Source: CAD feature listing. Evaluate the final solid. Frame: model axes, mm. Give positions to 0.01 mm unless a question says otherwise; leave off trailing zeros. Order: outer loops, then holes, each group sorted by start corner. A loop starts at its lowest first (then second) coordinate and runs counter-clockwise, first axis right, second up. Notation, with made-up numbers: M 69.5,62.25 L 126.5,62.25 A12 ccw 126.5,72.25 Z; hole C -26,52.5 d2. An arc over 180 degrees is marked long. Return JSON: item names as keys, results as strings.
from build123d import *

# Parameters (mm, degrees)
F0_W     = 266.7
F0_H     = 330.2
F1_DEPTH = 5.842
F2_W     = 266.7
F2_H     = 330.2
F2_W_2   = 215.9
F2_H_2   = 279.4
F3_DEPTH = 5.842
F6_R     = 9.525
F7_DEPTH = 11.685


with BuildPart() as f1:
    # F0 (on Front) → F1 (new body)
    with BuildSketch(Plane.XZ):
        with Locations((133.35, 165.1)):
            Rectangle(F0_W, F0_H)
    extrude(amount=F1_DEPTH)


with BuildPart() as f3:
    # F2 (on face) → F3 (new body)
    with BuildSketch(Plane.XZ.offset(5.842)):
        with Locations((133.35, 165.1)):
            Rectangle(F2_W, F2_H)
        with Locations((133.35, 165.1)):
            Rectangle(F2_W_2, F2_H_2, mode=Mode.SUBTRACT)
    extrude(amount=F3_DEPTH)


with BuildPart() as f1_1:
    add(f1.part)

    # F4: union F3
    add(f3.part)

    # F6 (on face) → F7 (cut, through all)
    with BuildSketch(Plane.XZ.offset(11.684)):
        with Locations((241.3, 304.8)):
            Circle(F6_R)
        with Locations((240.601733, 25.828205)):
            Circle(F6_R)
    extrude(amount=-F7_DEPTH, mode=Mode.SUBTRACT)


solid = f1_1.part
1. Section query B-B (x = 246). Return loops of the section in (y, z), then the cut area to 3 significant figures.
Evaluation:
{"outline": "M -11.68,0 L 0,0 L 0,17.98 L -11.68,17.98 Z; M -11.68,33.68 L 0,33.68 L 0,296.52 L -11.68,296.52 Z; M -11.68,313.08 L 0,313.08 L 0,330.2 L -11.68,330.2 Z", "area": "3,480 mm^2"}
2. Ray query, probe 1 along Z at (x, y) = (241.3, -4) (3 decimals); probe 2 along Z at (x, y) = (219.5, -7); probe 3 along X at (y, z) = (-6.75, 234). Return the intervals inside material, ascending.
Evaluation:
{"probe 1": "z = 0 to 16.329, 35.328 to 295.275, 314.325 to 330.2", "probe 2": "z = 0 to 25.4, 304.8 to 330.2", "probe 3": "x = 0 to 25.4, 241.3 to 266.7"}
3. Section query D-D (x = 137.5). Return loops of the section in (y, z), then the cut area to 3 significant figures.
Evaluation:
{"outline": "M -11.68,0 L 0,0 L 0,330.2 L -11.68,330.2 L -11.68,304.8 L -5.84,304.8 L -5.84,25.4 L -11.68,25.4 Z", "area": "2,230 mm^2"}
4. First-contact query: pin 1 (8 mm diameter, centred on x = 144, z = 179.5, fed in from -Y). Flat tip, straight axial feed; report the tip coordinate or a pass-through.
Evaluation:
{"pin 1": "stops at y = -5.84"}
5. Draft query along Z for faces 1 (the face through (13, -11.684, 167)), 2 (the face through (132, -5.842, 167)), 3 (the face through (131, -6, 0)). Return one class per face: pulls with the +Z half, pulls with the -Z half, needs draft (parallel to the pull), parting line crosses it, or undercut.
Evaluation:
{"face 1": "needs draft", "face 2": "undercut", "face 3": "pulls with the -Z half"}
6. Section query C-C (z = 244). Return loops of the section in (x, y), then the cut area to 3 significant figures.
Evaluation:
{"outline": "M 0,-11.68 L 25.4,-11.68 L 25.4,-5.84 L 241.3,-5.84 L 241.3,-11.68 L 266.7,-11.68 L 266.7,0 L 0,0 Z", "area": "1,850 mm^2"}
7. Section query A-A (y = -8.25). Return loops of the section in (x, z) (3 decimals), then the cut area to 3 significant figures.
Evaluation:
{"outline": "M 0,0 L 266.7,0 L 266.7,330.2 L 0,330.2 Z; hole M 25.4,25.4 L 231.086,25.4 A9.525 ccw long 241.3,35.328 L 241.3,295.275 A9.525 ccw long 231.775,304.8 L 25.4,304.8 Z", "area": "27,300 mm^2"}
